```python
from build123d import *

# Parameters (mm, degrees)
F0_R      = 64.5594783813
F1_DEPTH  = 1.524
F2_R      = 64.5594783813
F2_R_2    = 61.0323113023
F3_DEPTH  = 1.016
F4_R      = 16.6175214607
F5_DEPTH  = 16.764
F6_R      = 16.5608
F7_R      = 61.0868628562
F8_DEPTH  = 1.016
F13_W     = 3.8755843416
F13_H     = 16.3549613208
F13_W_2   = 3.6430479959
F14_DEPTH = 11.7094
F15_W     = 10.4532966083
F15_H     = 12.4406219693
F16_DEPTH = 37.6174


# Not quite as in the source:
# - the program builds the solid bodies; features that only make, move or delete a surface that nothing else refers to are left out


with BuildPart() as f1:
    # F0 (on Front) → F1 (new body, symmetric)
    with BuildSketch(Plane.XZ):
        Circle(F0_R)
    extrude(amount=F1_DEPTH, both=True)

    # F2 (on face) → F3 (join)
    with BuildSketch(Plane.XZ.offset(1.524)):
        Circle(F2_R)
        Circle(F2_R_2, mode=Mode.SUBTRACT)
    extrude(amount=F3_DEPTH)

    # F4 (on face) → F5 (join)
    with BuildSketch(Plane.XZ.offset(1.524)):
        Circle(F4_R)
    extrude(amount=F5_DEPTH)

    # F6
    f6_edges = [f1.edges().sort_by_distance(p)[0] for p in [
        (-16.617521, -18.288, 0),
    ]]
    fillet(f6_edges, radius=F6_R)

    # F7 (on face) → F8 (join)
    with BuildSketch(Plane(origin=(0, 1.524, 0), x_dir=(-1, 0, 0), z_dir=(0, 1, 0))):
        Circle(F7_R)
    extrude(amount=F8_DEPTH)

    # F13 (on face) → F14 (join)
    with BuildSketch(Plane(origin=(0, 2.54, 0), x_dir=(-1, 0, 0), z_dir=(0, 1, 0))):
        with Locations((-13.9141972177, -4.206892103)):
            Rectangle(F13_W, F13_H)
        with Locations((16.1215732805, -4.206892103)):
            Rectangle(F13_W_2, F13_H)
    extrude(amount=F14_DEPTH)

    # F15 (on face) → F16 (cut)
    with BuildSketch(Plane(origin=(-17.9430972785, 0, 0), x_dir=(0, -1, 0), z_dir=(-1, 0, 0))):
        with Locations((-7.7666483042, -4.7159082606)):
            Rectangle(F15_W, F15_H)
    extrude(amount=-F16_DEPTH, mode=Mode.SUBTRACT)


solid = f1.part
```
The listing builds one solid part. Answer for the finished solid, in the listing's coordinates (mm). A direction names the side the tool comes from. Give positions to 0.01 mm unless a question says otherwise; leave off trailing zeros. Order: outer loops, then holes, each group sorted by start corner. A loop starts at its lowest first (then second) coordinate and runs counter-clockwise, first axis right, second up. Notation, with made-up numbers: (35.5, 6) - (80.5, 6) arc R19 ccw to (80.5, 29) - close; hole circle Ø4 at (87.5, 25). An arc over 180 degrees is marked (long way). Answer in a Markdown table with one row per item. Add a question column.
Q1. The part is cut by section B-B (x = -56). Determine the outline of the cut face in (y, z), then the cut area to 3 significant figures.
Q2. The part is cut by section A-A (z = 20). Determine the outline of the cut face in (x, y), then the cut area to 3 significant figures.
Q3. Find the intervals of material crossed by line 1 along Z through (x, y) = (0, -2); line 2 along Y through (x, z) = (-8.5, -23.5); line 3 along Y through (x, z) = (4.5, -9), in increasing order. Write a range as [from, to].
Q4. Which of the six approach directions +Z, -Z, +X, -X, +Y, -Y give full straight-line access (tool end or side, diameter ignored) to faces 4 (the flat face through (-16, 8, -10.936)), 5 (the flat face through (-17.943, 14, -2)), 6 (the cylindrical face through (13.242, 2.025, -59.634))?
Q5. For a pull along X with two mould halves and no side action, classify faces 1 (the flat face through (15.852, 14, -2)), 2 (the flat face through (-16, 14.249, -4)), 3 (the flat face through (13, -1.524, -13)) as released by +X, released by -X, zero draft, split by the parting line, or undercut.
Q6. Given P1, Ø5, axis at y = 1, z = 6, coming from the -X side; P2, Ø8, axis at x = 3, y = -14.5, coming from the -Z side; P3, Ø13, axis at y = 10, z = -1, coming from the -X side, each flat-ended and moving along its own axis, determine where each tip first touches the part or whether it passes through.
Determined:
| question | item | result |
|---|---|---|
| 1 | outline | (-2.54, -32.12) - (1.52, -32.12) - (1.52, -24.41) - (2.54, -24.41) - (2.54, 24.41) - (1.52, 24.41) - (1.52, 32.12) - (-2.54, 32.12) - (-2.54, 24.27) - (-1.52, 24.27) - (-1.52, -24.27) - (-2.54, -24.27) - close |
| 1 | area | 261 mm² |
| 2 | outline | (-61.38, -2.54) - (-57.66, -2.54) - (-57.66, -1.52) - (57.66, -1.52) - (57.66, -2.54) - (61.38, -2.54) - (61.38, 1.52) - (57.72, 1.52) - (57.72, 2.54) - (-57.72, 2.54) - (-57.72, 1.52) - (-61.38, 1.52) - close |
| 2 | area | 499 mm² |
| 3 | line 1 | z = [-64.56, -61.03], [-16.62, 16.62], [61.03, 64.56] |
| 3 | line 2 | y = [-1.52, 2.54] |
| 3 | line 3 | y = [-14.92, 2.54] |
| 4 | face 4 | +X, -X |
| 4 | face 5 | +Z, -Z, -X, +Y |
| 4 | face 6 | +Y |
| 5 | face 1 | released by +X |
| 5 | face 2 | zero draft |
| 5 | face 3 | undercut |
| 6 | P1 | stops at x = -64.46 |
| 6 | P2 | stops at z = -13.88 |
| 6 | P3 | stops at x = -17.94 |
